Model file for the job. Use its own axes, mm. Face numbers are marked on the shaded views. Coordinates: 2 decimals unless noted, no trailing zeros. Write each loop counter-clockwise with the first axis right and the second up, starting at its lowest first coordinate (ties: lowest second). Pieces come first, ordered by that corner, then holes.
Q1. Band-saw the part on B-B, the plane y = -20. Write the cut outline in (x, z), plus the area to 3 significant figures.
Q2. Pin check, flat tips, straight feed: P1, Ø4.5, axis at x = 0, y = -20, coming from the +Z side; P2, Ø1.5, axis at x = 0.5, z = 49, coming from the -Y side. Stop position of each tip, or through.
Q3. Band-saw the part on A-A, the plane x = 0. Write the cut outline in (y, z), plus the area to 3 significant figures.
Q4. Drill centre lines: probe 1 along X at (y, z) = (-20, 51.05); probe 2 along X at (y, z) = (-20, 49.1); probe 3 along X at (y, z) = (-34.5, 48.35). Where is each one in solid material? Low to high.
Q5. Band-saw the part on C-C, the plane z = 49.8. Write the cut outline in (x, y), plus the area to 3 significant figures.
Q6. Pull direction Y, two halves, no side cores. Call the marked faces 1 and 2: released by +Y, released by -Y, zero draft, split by the parting line, or undercut.
from build123d import *

# Parameters (mm, degrees)
TORUS002_R        = 1.5
BOX084016_W       = 10
BOX084016_H       = 10
BOX084016_DEPTH   = 12
CYLINDER028_R     = 1.9
CYLINDER028_DEPTH = 10
CYLINDER012_R     = 18
CYLINDER012_DEPTH = 4


with BuildPart() as torus002:
    # Torus002 → Torus002 (revolve)
    with BuildSketch(Plane(origin=(0, 0, 2), x_dir=(1, 0, 0), z_dir=(0, -1, 0))):
        with Locations((19, 0)):
            Circle(TORUS002_R)
    revolve(axis=Axis((0, 0, 2), (0, 0, 1)))


with BuildPart() as cube067:
    # Box084016 → Box084016 (new body)
    with BuildSketch(Plane(origin=(-5, 1.1, -1.5), x_dir=(1, 0, 0), z_dir=(0, 0, 1))):
        with Locations((5, 5)):
            Rectangle(BOX084016_W, BOX084016_H)
    extrude(amount=BOX084016_DEPTH)


with BuildPart() as cut057:
    # Cylinder028 → Cylinder028 (new body)
    with BuildSketch(Plane.XY.offset(-1)):
        Circle(CYLINDER028_R)
    extrude(amount=CYLINDER028_DEPTH)

    # Cut057: cut Cube067
    add(cube067.part, mode=Mode.SUBTRACT)


with BuildPart() as wheel:
    # Cylinder012 → Cylinder012 (new body)
    with BuildSketch(Plane.XY):
        Circle(CYLINDER012_R)
    extrude(amount=CYLINDER012_DEPTH)

    # Cut062: cut Cut057
    add(cut057.part, mode=Mode.SUBTRACT)

    # Cut063: cut Torus002
    add(torus002.part, mode=Mode.SUBTRACT)


with BuildPart() as wheel_1:
    # Cut063 placement: moved
    add(wheel.part.moved(Location((0, -20, 48))))


solid = wheel_1.part
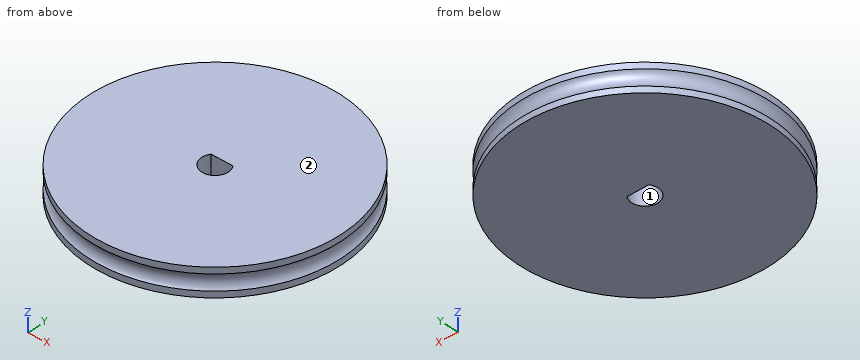
Answer sheet:
1. outline: (-18, 48) - (-1.9, 48) - (-1.9, 52) - (-18, 52) - (-18, 51.12) arc R1.5 cw to (-18, 48.88) - close; (1.9, 48) - (18, 48) - (18, 48.88) arc R1.5 cw to (18, 51.12) - (18, 52) - (1.9, 52) - close
1. area: 127 mm2
2. P1: stops at z = 52
2. P2: stops at y = -38
3. outline: (-38, 48) - (-21.9, 48) - (-21.9, 52) - (-38, 52) - (-38, 51.12) arc R1.5 cw to (-38, 48.88) - close; (-18.9, 48) - (-2, 48) - (-2, 48.88) arc R1.5 cw to (-2, 51.12) - (-2, 52) - (-18.9, 52) - close
3. area: 130 mm2
4. probe 1: x = -17.93 to -1.9, 1.9 to 17.93
4. probe 2: x = -17.8 to -1.9, 1.9 to 17.8
4. probe 3: x = -10.67 to 10.67
5. outline: circle Ø35.03 at (0, -20); hole (-1.55, -18.9) arc R1.9 ccw (long way) to (1.55, -18.9) - close
5. area: 954 mm2
6. face 1: undercut
6. face 2: zero draft
